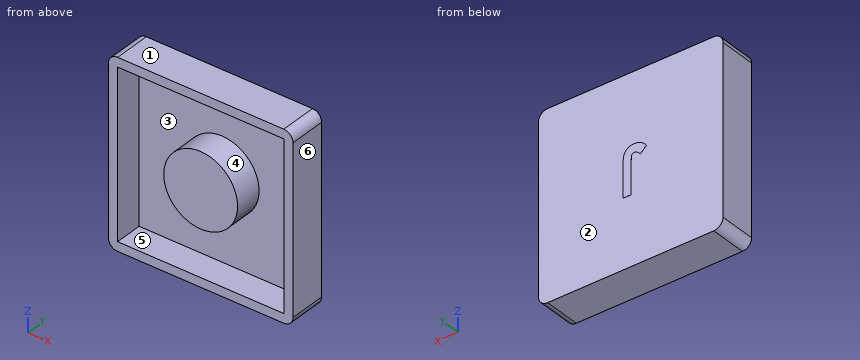
from build123d import *

# Parameters (mm, degrees)
SKETCH1_W           = 12.7
SKETCH1_H           = 12.7
BOSS_EXTRUDE1_DEPTH = 2.54
FILLET1_R           = 0.635
SHELL1_START        = 0.635
SHELL1_OUTLINE_W    = 1.905
SHELL1_OUTLINE_H    = 11.43
SHELL1_DEPTH        = 11.43
SKETCH2_R           = 2.54
BOSS_EXTRUDE2_DEPTH = 1.905
BOSS_EXTRUDE3_DEPTH = 0.00254


# Read off the part's stored shape, not the designer's step: Shell1
with BuildPart() as part:
    # Sketch1 → Boss-Extrude1 (new body)
    with BuildSketch(Plane(origin=(0, 0, 0), x_dir=(1, 0, 0), z_dir=(0, 1, 0))):
        with Locations((6.35, 6.35)):
            Rectangle(SKETCH1_W, SKETCH1_H)
    extrude(amount=BOSS_EXTRUDE1_DEPTH)

    # Fillet1
    fillet1_edges = [part.edges().sort_by_distance(p)[0] for p in [
        (0, 1.27, -12.7),
        (12.7, 1.27, -12.7),
        (12.7, 1.27, 0),
        (0, 1.27, 0),
    ]]
    fillet(fillet1_edges, radius=FILLET1_R)

    # Shell1 outline → Shell1 (cut)
    with BuildSketch(Plane.YZ.offset(SHELL1_START)):
        with Locations((0.9525, -6.35)):
            Rectangle(SHELL1_OUTLINE_W, SHELL1_OUTLINE_H)
    extrude(amount=SHELL1_DEPTH, mode=Mode.SUBTRACT)

    # Sketch2 → Boss-Extrude2 (add)
    with BuildSketch(Plane(origin=(0, 1.905, 0), x_dir=(-1, 0, 0), z_dir=(0, -1, 0))):
        with Locations(Location((-6.35, 6.35, 0), (0, 0, 270))):
            Circle(SKETCH2_R)
    extrude(amount=BOSS_EXTRUDE2_DEPTH)

    # Sketch3 → Boss-Extrude3 (add)
    with BuildSketch(Plane(origin=(0, 2.54, 0), x_dir=(1, 0, 0), z_dir=(0, 1, 0))):
        with BuildLine():
            Line((6.311248718, 8.001), (6.881120513, 8.001))
            Line((6.881120513, 8.001), (6.881120513, 5.89323758))
            add(Edge.make_bspline(
                [(6.881120513, 5.89323758), (6.880911581, 5.85295254), (6.88050901, 5.775331222), (6.876478561, 5.663585177), (6.871028683, 5.561130731), (6.863180334, 5.468132049), (6.851523386, 5.384593628), (6.83833126, 5.310307047), (6.823776683, 5.24496961), (6.799190432, 5.171846852), (6.76102099, 5.090871717), (6.703422211, 5.003407063), (6.631693296, 4.927415182), (6.549085279, 4.861407451), (6.454902126, 4.809141814), (6.351313596, 4.771364071), (6.238650837, 4.748795386), (6.160617709, 4.746019084), (6.120443429, 4.744589744)],
                knots=[0, 0, 0, 0, 1.22248561, 2.355488409, 3.392943897, 4.335991845, 5.186735882, 5.951517034, 6.625683685, 7.215700098, 8.28923535, 9.333114649, 10.380102123, 11.447198135, 12.530158036, 13.633358744, 14.781567393, 16, 16, 16, 16], degree=3))
            add(Edge.make_bspline(
                [(6.120443429, 4.744589744), (6.078585486, 4.745885617), (5.996025276, 4.748441587), (5.874942226, 4.77021188), (5.758566278, 4.80511621), (5.647499501, 4.855583683), (5.540220246, 4.918801011), (5.438675534, 4.997215953), (5.34074525, 5.088396519), (5.282691579, 5.158366196), (5.252915385, 5.194254207)],
                knots=[0, 0, 0, 0, 0.990984786, 1.954608977, 2.90473533, 3.862451285, 4.837525908, 5.848096122, 6.896271184, 8, 8, 8, 8], degree=3))
            Line((5.252915385, 5.194254207), (5.684135337, 5.59303726))
            add(Edge.make_bspline(
                [(5.684135337, 5.59303726), (5.706713527, 5.567507703), (5.74896339, 5.519735039), (5.812632688, 5.457438312), (5.870065826, 5.407390082), (5.924206265, 5.371289844), (5.975297298, 5.345843205), (6.024438185, 5.327513276), (6.073160718, 5.317137495), (6.105348309, 5.315340023), (6.121079447, 5.314461538)],
                knots=[0, 0, 0, 0, 1.529509877, 2.862124173, 3.996688592, 4.944357383, 5.774364335, 6.554177287, 7.293378699, 8, 8, 8, 8], degree=3))
            add(Edge.make_bspline(
                [(6.121079447, 5.314461538), (6.136305438, 5.315255549), (6.165580013, 5.316782171), (6.205833677, 5.333752509), (6.239770106, 5.360396654), (6.262111848, 5.391027555), (6.27634945, 5.422340582), (6.285245372, 5.452609437), (6.293687618, 5.48889359), (6.300451357, 5.531174856), (6.30556205, 5.580004736), (6.308109361, 5.634790439), (6.311207218, 5.695828017), (6.311234393, 5.738468063), (6.311248718, 5.760945913)],
                knots=[0, 0, 0, 0, 1.003927327, 1.930222208, 2.840933547, 3.835773585, 4.407906147, 5.114514582, 5.922289074, 6.876303333, 7.950072246, 9.174518422, 10.510537432, 12, 12, 12, 12], degree=3))
            Line((6.311248718, 5.760945913), (6.311248718, 8.001))
        make_face()
    extrude(amount=BOSS_EXTRUDE3_DEPTH)


solid = part.part
Here's how the part is built. I have some questions about the finished solid (model axes, mm). Face numbers are marked on the shaded views. A direction names the side the tool comes from. Coordinates: 2 decimals unless noted, no trailing zeros. Write each loop counter-clockwise with the first axis right and the second up, starting at its lowest first coordinate (ties: lowest second). Pieces come first, ordered by that corner, then holes.
1) If we section it at A-A (y = 0.4): List the corners of the cut face in (x, z) for me (3 decimals).
Filled in:
outline: (0, -12.065) arc R0.635 ccw to (0.635, -12.7) - (12.065, -12.7) arc R0.635 ccw to (12.7, -12.065) - (12.7, -0.635) arc R0.635 ccw to (12.065, 0) - (0.635, 0) arc R0.635 ccw to (0, -0.635) - close; circle Ø5.08 at (6.35, -6.35); hole (0.635, -12.065) - (12.065, -12.065) - (12.065, -0.635) - (0.635, -0.635) - close
2) Which directions (+Z, -Z, +X, -X, +Y, -Y) give clear straight access to the entire face, cutting with the end or side of a thin tool? Please do the marked faces 5 and 6.
Filled in:
face 5: -Y
face 6: +Z, -Z, +X, +Y, -Y
3) If we section it at D-D (z = -11.25): List the corners of the cut face in (x, y) for me (3 decimals), plus the area to 3 significant figures.
Filled in:
outline: (0, 0) - (0.635, 0) - (0.635, 1.905) - (12.065, 1.905) - (12.065, 0) - (12.7, 0) - (12.7, 2.54) - (0, 2.54) - close
area: 10.5 mm2
4) If I drill on line 1 (Z direction, x = 6.5, y = 0.35) (3 decimals); line 2 (Z direction, x = 2.5, y = 0.65) (3 decimals); line 3 (X direction, y = 0.25, z = -9) (3 decimals), over which ranges is the centre line in solid material (lowest first)?
Filled in:
line 1: z = -12.7 to -12.065, -8.886 to -3.814, -0.635 to 0
line 2: z = -12.7 to -12.065, -0.635 to 0
line 3: x = 0 to 0.635, 12.065 to 12.7
5) If we section it at C-C (x = 9.5): List the corners of the cut face in (y, z) for me (3 decimals).
Filled in:
outline: (0, -12.7) - (2.54, -12.7) - (2.54, 0) - (0, 0) - (0, -0.635) - (1.905, -0.635) - (1.905, -12.065) - (0, -12.065) - close
6) Thinking about a two-plate mould opening in Z: for the marked faces 1, 2, 3 and 4, which applies, +Z half, -Z half, draft (parallel to the pull), parting line (faces both ways), or undercut?
Filled in:
face 1: +Z half
face 2: draft
face 3: undercut
face 4: undercut
7) I'm going to push a flat-ended pin straight in: pin 1 (2 mm diameter, centred on x = 10.5, z = -7, fed in from -Y) (3 decimals). Where does the tip first touch, or does it pass through?
Filled in:
pin 1: stops at y = 1.905
